```python
from build123d import *

# Parameters (mm, degrees)
SKETCH_1_R          = 10
EXTRUDE_1_DEPTH     = 225
SKETCH_2_R          = 15
EXTRUDE_2_DEPTH     = 5
CUT_EXTRUDE_1_DEPTH = 18
FILLET_1_R          = 1


with BuildPart() as part:
    # 草图1 → 凸台-拉伸1 (new body)
    with BuildSketch(Plane.XY):
        Circle(SKETCH_1_R)
    extrude(amount=EXTRUDE_1_DEPTH)

    # 草图2 → 凸台-拉伸2 (add)
    with BuildSketch(Plane(origin=(0, 0, 110), x_dir=(-1, 0, 0), z_dir=(0, 0, -1))):
        Circle(SKETCH_2_R)
    extrude(amount=-EXTRUDE_2_DEPTH)

    # 草图4 → 切除-拉伸1 (cut)
    with BuildSketch(Plane(origin=(0, 7, 0), x_dir=(-1, 0, 0), z_dir=(0, 1, 0))):
        with BuildLine():
            Line((-2.5, 208.431386243), (-2.5, 218.431386243))
            ThreePointArc((-2.5, 218.431386243), (0, 220.931386243), (2.5, 218.431386243))
            Line((2.5, 218.431386243), (2.5, 208.431386243))
            ThreePointArc((2.5, 208.431386243), (0, 205.931386243), (-2.5, 208.431386243))
        make_face()
    extrude(amount=CUT_EXTRUDE_1_DEPTH, mode=Mode.SUBTRACT)

    # 圆角1
    fillet_1_edges = [part.edges().sort_by_distance(p)[0] for p in [
        (-10, 0, 225),
    ]]
    fillet(fillet_1_edges, radius=FILLET_1_R)


solid = part.part
```
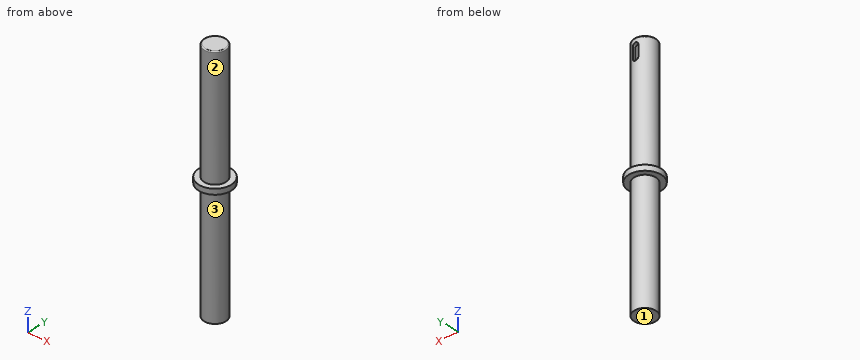
Geometry check sheet. Reference: the model listing, model coordinates, mm. Face numbers are marked on the shaded views. A direction names the side the tool comes from. Round coordinates to 2 decimals unless told otherwise and drop trailing zeros. Order: outer loops, then holes, each group sorted by start corner. A loop starts at its lowest first (then second) coordinate and runs counter-clockwise, first axis right, second up. Notation, with made-up numbers: M -35.75,-12 L 18.25,-12 A10 ccw 18.25,-4 Z; hole C -18,54 d3. An arc over 180 degrees is marked long. Answer as CSV lines item,"result".
1) Gauge pin test, flat ends, axial feed: pin 1 Ø12 at (y, z) = (9, 170.5) entering from +X; pin 2 Ø9 at (x, y) = (-2.5, 1.5) entering from -Z; pin 3 Ø6 at (x, z) = (5, 83.5) entering from -Y; pin 4 Ø2 at (y, z) = (8, 212.5) entering from -X. Record the tip position at first contact, or that the pin passes through.
Entries:
pin 1,"x = 9.54"
pin 2,"z = 0"
pin 3,"y = -9.8"
pin 4,"x = -7.14"
2) Sectioned sample at C-C on z = 179.5. Record the cut outline in (x, y).
Entries:
outline,"C 0,0 d20"
3) Tool access check on the marked faces 1, 2 and 3. Record the directions out of +Z, -Z, +X, -X, +Y, -Y that give a thin tool (end or side, any length) a straight path to the whole face; none if there is none.
Entries:
face 1,"-Z, +X, -X, +Y, -Y"
face 2,"+Z"
face 3,"-Z"
4) Thickness scan on probe 1 along X at (y, z) = (0.75, 99); probe 2 along Z at (x, y) = (-10.25, -6); probe 3 along Y at (x, z) = (-0.5, 189.5). Record the ranges inside material, lowest first. Write a range as [from, to].
Entries:
probe 1,"[-9.97, 9.97]"
probe 2,"[110, 115]"
probe 3,"[-9.99, 9.99]"
5) Sectioned sample at A-A on y = 0. Record the cut outline in (x, z), and give its area (3 significant figures).
Entries:
outline,"M -15,110 L -10,110 L -10,0 L 10,0 L 10,110 L 15,110 L 15,115 L 10,115 L 10,224 A1 ccw 9,225 L -9,225 A1 ccw -10,224 L -10,115 L -15,115 Z"
area,"4,550 mm2"
6) Sectioned sample at D-D on x = -13. Record the cut outline in (y, z), and give its area (3 significant figures).
Entries:
outline,"M -7.48,110 L 7.48,110 L 7.48,115 L -7.48,115 Z"
area,"74.8 mm2"
7) Sectioned sample at B-B on x = 0. Record the cut outline in (y, z), and give its area (3 significant figures).
Entries:
outline,"M -15,110 L -10,110 L -10,0 L 10,0 L 10,110 L 15,110 L 15,115 L 10,115 L 10,205.93 L 7,205.93 L 7,220.93 L 10,220.93 L 10,224 A1 ccw 9,225 L -9,225 A1 ccw -10,224 L -10,115 L -15,115 Z"
area,"4,500 mm2"
